Geometry: final body of the model. Coordinates: model frame, mm. Face numbers are marked on the shaded views. Give positions to 0.01 mm unless a question says otherwise; leave off trailing zeros. Loops run counter-clockwise (first coordinate to the right, second up) from the corner with the lowest first, then second, coordinate; pieces in that order, holes last. Notation, with made-up numbers: (82, -3.75) -> (86, -3.75) arc R29 ccw to (86, 30.25) -> close; hole circle Ø7 at (61, 38.5). An arc over 180 degrees is marked (long way). Answer in a Markdown table with one row per item. Add a question column.
Autodesk Inventor part; units mm, degrees
ref_plane "XZ Plane" through (0, 0, 0) normal (0, 1, 0) x (-1, 0, 0)
ref_plane "XY Plane" through (0, 0, 0) normal (0, 0, 1) x (1, 0, 0)
sketch "Sketch1" plane through (0, 0, 0) normal (0, 0, 1) x (1, 0, 0)
  line L0 (-62.23, 32.385) -> (62.23, 32.385)
  line L1 (62.23, -32.385) -> (-62.23, -32.385)
  line L2 (62.23, 0) -> (68.58, 0) construction
  line L3 (-62.23, 0) -> (-68.58, 0) construction
  ellipse E0 centre (-62.23, 0) end of major axis (-68.58, 0) minor radius 32.385 (-62.23, 32.385) -> (-62.23, -32.385) ccw
  ellipse E1 centre (62.23, 0) end of major axis (68.58, 0) minor radius 32.385 (62.23, -32.385) -> (62.23, 32.385) ccw
  point P0 (0, 0)
  dimension "d2" = 64.77
  dimension "d3" = 32.385
  dimension "d4" = 6.35
  dimension "d5" = 6.35
  dimension "d6" = 62.23
  dimension "d7" = 68.58
extrude "Extrusion1" add sketch "Sketch1" along normal blind 16.256
ref_plane "Work Plane1" through (-68.58, 0, 0) normal (1, 0, 0) x (0, 1, 0)
sketch "Sketch2" plane through (0, 0, 0) normal (1, 0, 0) x (0, 1, 0)
  point P0 (0, 0)
sketch "Sketch3" plane through (-68.58, 0, 0) normal (1, 0, 0) x (0, 1, 0)
  circle A0 centre (-15.5448, 4.1402) radius 1.6002
  line L0 (-32.385, 0) -> (32.385, 0)
  line L1 (-32.385, 0) -> (-32.385, 16.256)
  point P0 (0, 0)
  dimension "d10" = 3.2004
  dimension "d11" = 2.54
  dimension "d12" = 15.24
extrude "Extrusion2" cut sketch "Sketch3" along normal blind 9.525
sketch "Sketch4" plane through (-68.58, 0, 0) normal (1, 0, 0) x (0, 1, 0)
  line L0 (3.937, 2.794) -> (-6.985, 2.794)
  line L1 (-6.985, 2.794) -> (-6.985, 6.223)
  line L2 (-6.985, 6.223) -> (3.937, 6.223)
  line L3 (3.937, 6.223) -> (3.937, 2.794)
  line L4 (-32.385, 0) -> (32.385, 0)
  line L5 (-32.385, 0) -> (-32.385, 16.256)
  point P0 (0, 0)
  dimension "d15" = 3.429
  dimension "d16" = 10.922
  dimension "d17" = 2.794
  dimension "d18" = 25.4
extrude "Extrusion3" cut sketch "Sketch4" along normal blind 2.54
sketch "Sketch5" plane through (0, 0, 16.256) normal (0, 0, 1) x (1, 0, 0)
  line L0 (-62.23, 32.385) -> (62.23, 32.385)
  line L1 (-58.42, 26.1874) -> (28.448, 26.1874)
  line L2 (28.448, 26.1874) -> (28.448, -24.6126)
  line L3 (28.448, -24.6126) -> (-58.42, -24.6126)
  line L4 (-58.42, -24.6126) -> (-58.42, 26.1874)
  point P0 (0, 0)
  dimension "d21" = 50.8
  dimension "d22" = 86.868
  dimension "d23" = 3.81
  dimension "d24" = 6.1976
extrude "Extrusion4" cut sketch "Sketch5" against normal blind 1.27
properties part number "SprintSamsungGalaxyS"
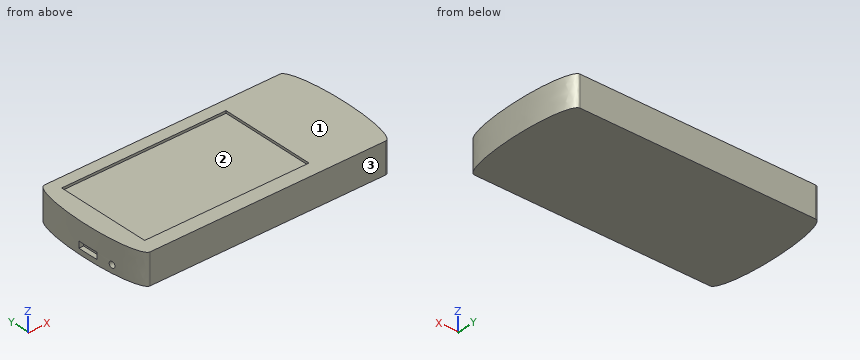
(1) Draft query along Y for the marked faces 1, 2 and 3. Return one class per face: +Y half, -Y half, draft (parallel to the pull), parting line (faces both ways), or undercut.
(2) Cut plane A-A on x = -4. Return the cut outline in (y, z) (3 decimals).
(3) Material intervals for line 1 along X through (y, z) = (-1, 9.25); line 2 along Z through (x, y) = (-18.5, 21); line 3 along X through (y, z) = (-13, 6.5), sorted ascending. Write a range as from..to.
(4) Pin query (flat end, axial travel): pin 1 Ø2 at (x, y) = (-36.5, 1.5) entering from +Z; pin 2 Ø2.5 at (y, z) = (-3, 4) entering from -X; pin 3 Ø0.6 at (y, z) = (8, 15.5) entering from +X. Return the tip coordinate at first contact, or that it passes through.
Answer list:
| question | item | result |
|---|---|---|
| 1 | face 1 | draft |
| 1 | face 2 | undercut |
| 1 | face 3 | -Y half |
| 2 | outline | (-32.385, 0) -> (32.385, 0) -> (32.385, 16.256) -> (26.187, 16.256) -> (26.187, 14.986) -> (-24.613, 14.986) -> (-24.613, 16.256) -> (-32.385, 16.256) -> close |
| 3 | line 1 | x = -68.58..68.58 |
| 3 | line 2 | z = 0..14.99 |
| 3 | line 3 | x = -68.05..68.05 |
| 4 | pin 1 | stops at z = 14.99 |
| 4 | pin 2 | stops at x = -68.56 |
| 4 | pin 3 | stops at x = 68.4 |
